```python
from build123d import *

# Parameters (mm, degrees)
CUT_EXTRUDE_1_DEPTH      = 29.955396734
CUT_EXTRUDE_1_DEPTH_BACK = 29.955396734
SKETCH_2_R               = 1.55
CHAMFER_1_SIZE           = 0.5
SKETCH_4_R               = 5.3
SKETCH_4_R_2             = 2.1
EXTRUDE_1_DEPTH          = 3
SKETCH_5_R               = 1.5
CUT_EXTRUDE_2_DEPTH      = 19
CUT_EXTRUDE_3_DEPTH      = 38


with BuildPart() as part:
    # 草图1 → 旋转1 (revolve)
    with BuildSketch(Plane.XY, mode=Mode.PRIVATE) as revolve_1_sk:
        Polygon((5.3, -24.9), (5.3, 15.1), (10.45, 15.1), (10.45, 10.1), (7.45, 10.1), (7.45, -24.9), align=None)
    revolve(revolve_1_sk.sketch.rotate(Axis((0, 0, 0), (0, 1, 0)), 90), axis=Axis((0, 0, 0), (0, 1, 0)))

    # 草图2 → 切除-拉伸1 (cut, two sides: drawn at the far end of the back side and taken through both)
    with BuildSketch(Plane.XY.offset(-CUT_EXTRUDE_1_DEPTH_BACK)):
        with Locations((0, -15.9)):
            Circle(SKETCH_2_R)
    extrude(amount=CUT_EXTRUDE_1_DEPTH + CUT_EXTRUDE_1_DEPTH_BACK, mode=Mode.SUBTRACT)

    # 倒角1
    chamfer_1_edges = [part.edges().sort_by_distance(p)[0] for p in [
        (0, -24.9, 7.45),
    ]]
    chamfer(chamfer_1_edges, length=CHAMFER_1_SIZE)

    # 草图3 → 旋转2 (revolve)
    with BuildSketch(Plane(origin=(0, 0, 0), x_dir=(0, 0, -1), z_dir=(1, 0, 0)), mode=Mode.PRIVATE) as revolve_2_sk:
        Polygon((10.45, 15.1), (15.1, 15.1), (15.1, 10.6), (13.1, 10.6), (13.1, 13.1), (10.409558261, 13.1), (10.409558261, 15.1), align=None)
    revolve(revolve_2_sk.sketch.rotate(Axis((0, 0, 0), (0, -1, 0)), 180), axis=Axis((0, 0, 0), (0, -1, 0)))

    # 草图4 → 凸台-拉伸1 (add)
    with BuildSketch(Plane(origin=(0, 15.1, 0), x_dir=(1, 0, 0), z_dir=(0, 1, 0))):
        with Locations(Location((0, 0, 0), (0, 0, 90))):
            Circle(SKETCH_4_R)
        with Locations(Location((0, 0, 0), (0, 0, 270))):
            Circle(SKETCH_4_R_2, mode=Mode.SUBTRACT)
    extrude(amount=-EXTRUDE_1_DEPTH)

    # 草图5 → 切除-拉伸2 (cut)
    with BuildSketch(Plane.XZ.offset(-10.1)):
        with Locations(Location((-8.449926035, 8.449926035, 0), (0, 0, 315))):
            Circle(SKETCH_5_R)
        with Locations(Location((8.449926035, 8.449926035, 0), (0, 0, 225))):
            Circle(SKETCH_5_R)
        with Locations(Location((8.449926035, -8.449926035, 0), (0, 0, 272.799179687))):
            Circle(SKETCH_5_R)
        with Locations(Location((-8.449926035, -8.449926035, 0), (0, 0, 267.200820313))):
            Circle(SKETCH_5_R)
    extrude(amount=-CUT_EXTRUDE_2_DEPTH, mode=Mode.SUBTRACT)

    # 草图7 → 切除-拉伸3 (cut)
    with BuildSketch(Plane.XZ.offset(24.9)):
        with BuildLine():
            Line((-3.229227591, 9.938540595), (-5.325886772, 16.39139404))
            ThreePointArc((-5.325886772, 16.39139404), (0, -17.234931636), (5.325886772, 16.39139404))
            Line((5.325886772, 16.39139404), (3.229227591, 9.938540595))
            ThreePointArc((3.229227591, 9.938540595), (0, -10.45), (-3.229227591, 9.938540595))
        make_face()
    extrude(amount=-CUT_EXTRUDE_3_DEPTH, mode=Mode.SUBTRACT)


solid = part.part
```
Read the model definition and answer for the solid it produces. Units are mm, in the model's axes. A direction names the side the tool comes from. Round coordinates to 2 decimals unless told otherwise and drop trailing zeros. Write each loop counter-clockwise with the first axis right and the second up, starting at its lowest first coordinate (ties: lowest second). Pieces come first, ordered by that corner, then holes. Notation, with made-up numbers: (84.5, -38) -> (102.5, -38) arc R23 ccw to (102.5, -15) -> close; hole circle Ø4 at (74.5, 86). An arc over 180 degrees is marked (long way). Answer in a Markdown table with one row per item. Add a question column.
1) Find section A-A, the plane z = 0. Determine the outline of the cut face in (x, y).
2) Find section D-D, the plane y = -15.9. Determine the outline of the cut face in (x, z), and give its area (3 significant figures).
3) Determine the mould class of faces 5 (the face through (-4.54, 13.82, 14.4)), 6 (the face through (3.22, -6.14, 4.21)), 7 (the face through (-1.23, -16.84, 6.24)) for opening direction Z: pulls with the +Z half, pulls with the -Z half, needs draft (parallel to the pull), parting line crosses it, or undercut.
4) Find section B-B, the plane x = 8. Determine the outline of the cut face in (y, z).
5) Find section C-C, the plane x = 0. State how many separate pieces and enclosed holes the cut face has, and give its area (3 significant figures).
6) Consider line 1 (Y direction, x = 0, z = 5.85); line 2 (Z direction, x = -8, y = 13.5); line 3 (X direction, y = -15.9, z = -6.25). Determine where each line is inside the solid, lowest interval first.
7) Which of the six approach directions +Z, -Z, +X, -X, +Y, -Y give full straight-line access (tool end or side, diameter ignored) to faces 1 (the face through (0, 10.6, 14)), 2 (the face through (4.36, 11.83, 13.42)), 3 (the face through (-2.238, -7.391, -7.106)), 4 (the face through (-4.353, 11.833, 13.397))?
8) Given P1, Ø3, axis at x = 0, z = 14, coming from the -Y side; P2, Ø4, axis at x = 0, y = -15.9, coming from the -Z side; P3, Ø6, axis at x = 11.5, y = 9.5, coming from the +Z side; P4, Ø1.8, axis at x = 8.45, z = 8.45, coming from the +Y side, each flat-ended and moving along its own axis, determine where each tip first touches the part or whether it passes through.
Findings below:
| question | item | result |
|---|---|---|
| 1 | outline | (-15.1, 13.1) -> (-10.45, 13.1) -> (-10.45, 10.1) -> (-7.45, 10.1) -> (-7.45, -24.4) -> (-6.95, -24.9) -> (-5.3, -24.9) -> (-5.3, 12.1) -> (-2.1, 12.1) -> (-2.1, 15.1) -> (-15.1, 15.1) -> close; (2.1, 12.1) -> (5.3, 12.1) -> (5.3, -24.9) -> (6.95, -24.9) -> (7.45, -24.4) -> (7.45, 10.1) -> (10.45, 10.1) -> (10.45, 13.1) -> (15.1, 13.1) -> (15.1, 15.1) -> (2.1, 15.1) -> close |
| 2 | outline | (-1.55, -7.29) -> (-1.55, -5.07) arc R5.3 cw to (-1.55, 5.07) -> (-1.55, 7.29) arc R7.45 ccw to start; (1.55, -7.29) arc R7.45 ccw to (1.55, 7.29) -> (1.55, 5.07) arc R5.3 cw to (1.55, -5.07) -> close |
| 2 | area | 72.6 mm² |
| 3 | face 5 | parting line crosses it |
| 3 | face 6 | undercut |
| 3 | face 7 | needs draft |
| 4 | outline | (10.1, -6.72) -> (13.1, -6.72) -> (13.1, -7.02) -> (15.1, -7.02) -> (15.1, 7.02) -> (13.1, 7.02) -> (13.1, 6.72) -> (10.1, 6.72) -> close; (13.1, -12.81) -> (15.1, -12.81) -> (15.1, -9.88) -> (13.1, -9.88) -> close; (13.1, 9.88) -> (15.1, 9.88) -> (15.1, 12.81) -> (13.1, 12.81) -> close |
| 5 | separate pieces | 4 |
| 5 | enclosed holes | 0 |
| 5 | area | 231 mm² |
| 6 | line 1 | -24.9 to -17.45, -14.35 to 15.1 |
| 6 | line 2 | -12.81 to -9.88, -7.02 to 7.02, 9.88 to 12.81 |
| 6 | line 3 | -4.05 to -1.55, 1.55 to 4.05 |
| 7 | face 1 | +Z, +X, -X, -Y |
| 7 | face 2 | +X, -Y |
| 7 | face 3 | -Y |
| 7 | face 4 | -X, -Y |
| 8 | P1 | y = 10.6 |
| 8 | P2 | z = -7.45 |
| 8 | P3 | z = 5.99 |
| 8 | P4 | through |
